Design review of the part shown in the three views and the two pictorial views. Dimensions are in mm from the part's minimum x, y and z. A direction names the side the tool comes from. Round coordinates to 2 decimals unless told otherwise and drop trailing zeros. Loops run counter-clockwise (first coordinate to the right, second up) from the corner with the lowest first, then second, coordinate; pieces in that order, holes last.
1) Tool access review of the marked faces 1, 2, 3, 4 and 5: name each direction out of +Z, -Z, +X, -X, +Y, -Y from which nothing blocks a thin tool from reaching the whole face with its end or side.
2) Take a section at B-B (x = 7). State the section outline as (y, z) points, then the cut area to 3 significant figures.
3) Mouldability with a two-part tool opening along X and no side actions: class the marked faces 6, 7, 8 and 9 as pulls with the +X half, pulls with the -X half, needs draft (parallel to the pull), parting line crosses it, or undercut.
4) Wall thickness on L1, parallel to X at y = 1, z = 2.5; L2, parallel to Z at x = 2.5, y = 1.1; L3, parallel to X at y = 10.25, z = 9: over which ranges is each line inside the solid? List them lowest first.
5) Insertion check: pin 1 (3.5 mm diameter, centred on y = 10, z = 15, fed in from -X); pin 2 (4 mm diameter, centred on x = 48.5, z = 23.5, fed in from +Y); pin 3 (3 mm diameter, centred on x = 34.5, y = 6.5, fed in from +Z). Each pin has a flat end and moves straight along its axis. Give the tip position at first contact, or say it passes through.
6) Take a section at A-A (y = 3.75). State the section outline as (x, z) points, then the cut area to 3 significant figures.
7) Take a section at C-C (z = 2.5). State the section outline as (x, y) points, then the cut area to 3 significant figures.
8) Take a section at D-D (x = 48.5). State the section outline as (y, z) points, then the cut area to 3 significant figures.
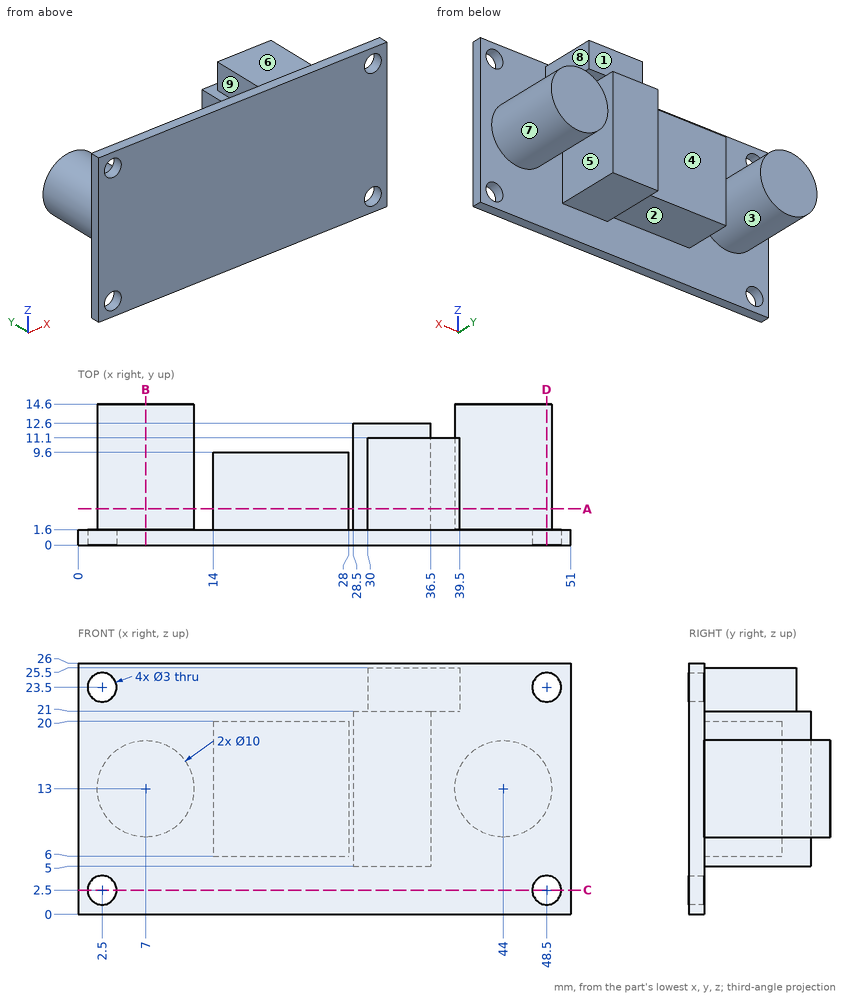
Response:
1. face 1: +Z, +X, -X, +Y
1. face 2: -Z, -X, +Y
1. face 3: +Y
1. face 4: +Z, -Z, +Y
1. face 5: -Z, +Y
2. outline: (0, 0) - (1.6, 0) - (1.6, 8) - (14.6, 8) - (14.6, 18) - (1.6, 18) - (1.6, 26) - (0, 26) - close
2. area: 172 mm2
3. face 6: needs draft
3. face 7: undercut
3. face 8: pulls with the +X half
3. face 9: pulls with the -X half
4. L1: x = 0 to 1, 4 to 47, 50 to 51
4. L2: z = 0 to 1, 4 to 22, 25 to 26
4. L3: x = 4 to 10, 28.5 to 36.5, 41 to 47
5. pin 1: stops at x = 2.01
5. pin 2: stops at y = 1.6
5. pin 3: stops at z = 25.5
6. outline: circle Ø10 at (7, 13); (14, 6) - (28, 6) - (28, 20) - (14, 20) - close; (28.5, 5) - (36.5, 5) - (36.5, 21) - (39.5, 21) - (39.5, 25.5) - (30, 25.5) - (30, 21) - (28.5, 21) - close; circle Ø10 at (44, 13)
6. area: 524 mm2
7. outline: (0, 0) - (1, 0) - (1, 1.6) - (0, 1.6) - close; (4, 0) - (47, 0) - (47, 1.6) - (4, 1.6) - close; (50, 0) - (51, 0) - (51, 1.6) - (50, 1.6) - close
7. area: 72.0 mm2
8. outline: (0, 0) - (1.6, 0) - (1.6, 1) - (0, 1) - close; (0, 4) - (1.6, 4) - (1.6, 10.82) - (14.6, 10.82) - (14.6, 15.18) - (1.6, 15.18) - (1.6, 22) - (0, 22) - close; (0, 25) - (1.6, 25) - (1.6, 26) - (0, 26) - close
8. area: 88.7 mm2
